Verification items for the finished model (mm, model axes). A direction names the side the tool comes from. Give positions to 0.01 mm unless a question says otherwise; leave off trailing zeros. Loops run counter-clockwise (first coordinate to the right, second up) from the corner with the lowest first, then second, coordinate; pieces in that order, holes last. Notation, with made-up numbers: (64, 9) - (120, 9) arc R15 cw to (120, 36) - close; hole circle Ø8 at (-31.5, -37.5). An arc over 180 degrees is marked (long way). Answer in a Markdown table with one row per item.
```python
from build123d import *

# Parameters (mm, degrees)
EXTRUDE_1_DEPTH     = 19
SKETCH_3_W          = 23.2
SKETCH_3_H          = 9
CUT_EXTRUDE_2_DEPTH = 31.8
CUT_EXTRUDE_3_DEPTH = 8
SKETCH_5_W          = 7.5
SKETCH_5_H          = 7.5
CUT_EXTRUDE_4_DEPTH = 31.8
SKETCH_6_R          = 1.4
CUT_EXTRUDE_5_DEPTH = 27
SKETCH_7_R          = 0.75
CUT_EXTRUDE_6_DEPTH = 31.8
FILLET_2_R          = 0.5
FILLET_3_R          = 2
FILLET_4_R          = 0.5


with BuildPart() as part:
    # 草图1 → 凸台-拉伸1 (new body)
    with BuildSketch(Plane(origin=(0, 0, 0), x_dir=(1, 0, 0), z_dir=(0, 1, 0))):
        Polygon((-5.22, 18.4025), (-2.42, 18.4025), (-2.42, -6.5975), (20.78, -6.5975), (20.78, -12.3975), (-5.22, -12.3975), align=None)
    extrude(amount=EXTRUDE_1_DEPTH)

    # 草图3 → 切除-拉伸2 (cut, through all)
    with BuildSketch(Plane.XY.offset(12.3975)):
        with Locations((9.18, 14.5)):
            Rectangle(SKETCH_3_W, SKETCH_3_H)
    extrude(amount=-CUT_EXTRUDE_2_DEPTH, mode=Mode.SUBTRACT)

    # 草图4 → 切除-拉伸3 (cut)
    with BuildSketch(Plane(origin=(0, 10, 0), x_dir=(1, 0, 0), z_dir=(0, 1, 0))):
        with BuildLine():
            Line((-0.82, -8.4975), (19.18, -8.4975))
            ThreePointArc((19.18, -8.4975), (20.18, -9.4975), (19.18, -10.4975))
            Line((19.18, -10.4975), (-0.82, -10.4975))
            ThreePointArc((-0.82, -10.4975), (-1.82, -9.4975), (-0.82, -8.4975))
        make_face()
    extrude(amount=-CUT_EXTRUDE_3_DEPTH, mode=Mode.SUBTRACT)

    # 草图5 → 切除-拉伸4 (cut, through all)
    with BuildSketch(Plane.XY.offset(12.3975)):
        with Locations((9.18, 6.25)):
            Rectangle(SKETCH_5_W, SKETCH_5_H)
    extrude(amount=-CUT_EXTRUDE_4_DEPTH, mode=Mode.SUBTRACT)

    # 草图6 → 切除-拉伸5 (cut, through all)
    with BuildSketch(Plane.ZY.offset(5.22)):
        with Locations((-16.4025, 17)):
            Circle(SKETCH_6_R)
        with Locations((4.5975, 17)):
            Circle(SKETCH_6_R)
        with Locations((-16.4025, 3.5)):
            Circle(SKETCH_6_R)
        with Locations((4.5975, 3.5)):
            Circle(SKETCH_6_R)
    extrude(amount=-CUT_EXTRUDE_5_DEPTH, mode=Mode.SUBTRACT)

    # 草图7 → 切除-拉伸6 (cut, through all)
    with BuildSketch(Plane.XY.offset(12.3975)):
        with Locations((2.88, 6.2)):
            Circle(SKETCH_7_R)
        with Locations((15.48, 6.2)):
            Circle(SKETCH_7_R)
    extrude(amount=-CUT_EXTRUDE_6_DEPTH, mode=Mode.SUBTRACT)

    # 圆角2
    fillet_2_edges = [part.edges().sort_by_distance(p)[0] for p in [
        (-5.22, 9.5, -18.4025),
        (-2.42, 9.5, -18.4025),
        (-5.22, 9.5, 12.3975),
    ]]
    fillet(fillet_2_edges, radius=FILLET_2_R)

    # 圆角3
    fillet_3_edges = [part.edges().sort_by_distance(p)[0] for p in [
        (20.78, 5, 6.5975),
        (20.78, 5, 12.3975),
    ]]
    fillet(fillet_3_edges, radius=FILLET_3_R)

    # 圆角4
    fillet_4_edges = [part.edges().sort_by_distance(p)[0] for p in [
        (-2.42, 14.5, 12.3975),
    ]]
    fillet(fillet_4_edges, radius=FILLET_4_R)


solid = part.part
```
Q1. Sectioned sample at D-D (z = 4). Record the cut outline in (x, y).
Completed:
| item | result |
|---|---|
| outline | (-5.22, 0) - (-2.42, 0) - (-2.42, 2.23) - (-5.22, 2.23) - close; (-5.22, 4.77) - (-2.42, 4.77) - (-2.42, 15.73) - (-5.22, 15.73) - close; (-5.22, 18.27) - (-2.42, 18.27) - (-2.42, 19) - (-5.22, 19) - close |
Q2. Go/stop test with flat-tipped pins: P1, Ø10, axis at x = 8, y = 9.5, coming from the -Z side; P2, Ø1, axis at x = 7.5, z = 8, coming from the +Y side; P3, Ø2, axis at x = 15.48, y = 6.2, coming from the +Z side; P4, Ø12, axis at x = 11.5, z = 8.5, coming from the +Y side. Record where each tip stops, or that it passes through.
Completed:
| item | result |
|---|---|
| P1 | z = 6.6 |
| P2 | y = 2.5 |
| P3 | z = 12.4 |
| P4 | y = 10 |
Q3. Sectioned sample at A-A (y = 3.5). Give the number of separate pieces and of enclosed holes in the cut face, and give its area (3 significant figures).
Completed:
| item | result |
|---|---|
| separate pieces | 4 |
| enclosed holes | 0 |
| area | 132 mm^2 |
Q4. Tool access check on faces 5 (the face through (8, 2, 6.598)), 6 (the face through (20.18, 6.06, 9.48)), 7 (the face through (9, 2.5, 11)). Record the directions out of +Z, -Z, +X, -X, +Y, -Y that give a thin tool (end or side, any length) a straight path to the whole face; none if there is none.
Completed:
| item | result |
|---|---|
| face 5 | -Z, +X, +Y, -Y |
| face 6 | +Y |
| face 7 | +Z, -Z, +Y |
Q5. Sectioned sample at C-C (x = 15.48). Record the cut outline in (y, z), and give its area (3 significant figures).
Completed:
| item | result |
|---|---|
| outline | (0, 6.6) - (5.45, 6.6) - (5.45, 8.5) - (2, 8.5) - (2, 10.5) - (5.45, 10.5) - (5.45, 12.4) - (0, 12.4) - close; (6.95, 6.6) - (10, 6.6) - (10, 8.5) - (6.95, 8.5) - close; (6.95, 10.5) - (10, 10.5) - (10, 12.4) - (6.95, 12.4) - close |
| area | 36.3 mm^2 |
Q6. Sectioned sample at B-B (y = 8). Record the cut outline in (x, z).
Completed:
| item | result |
|---|---|
| outline | (-5.22, -17.9) arc R0.5 ccw to (-4.72, -18.4) - (-2.92, -18.4) arc R0.5 ccw to (-2.42, -17.9) - (-2.42, 6.6) - (5.43, 6.6) - (5.43, 8.5) - (-0.82, 8.5) arc R1 cw to (-0.82, 10.5) - (5.43, 10.5) - (5.43, 12.4) - (-4.72, 12.4) arc R0.5 ccw to (-5.22, 11.9) - close; (12.93, 6.6) - (18.78, 6.6) arc R2 ccw to (20.78, 8.6) - (20.78, 10.4) arc R2 ccw to (18.78, 12.4) - (12.93, 12.4) - (12.93, 10.5) - (19.18, 10.5) arc R1 cw to (19.18, 8.5) - (12.93, 8.5) - close |
Q7. Thickness scan on line 1 (Y direction, x = 2.88, z = 7.8); line 2 (Z direction, x = 17.25, y = 8); line 3 (X direction, y = 6.25, z = -15.5). Record the ranges inside material, lowest first.
Completed:
| item | result |
|---|---|
| line 1 | 0 to 5.45, 6.95 to 10 |
| line 2 | 6.6 to 8.5, 10.5 to 12.4 |
| line 3 | -5.22 to -2.42 |
Q8. Draft check along Y on faces 1 (the face through (14.73, 6.23, 7.56)), 2 (the face through (-4, 19, -3)), 3 (the face through (20.18, 5.07, 7.17)), 4 (the face through (-3.84, 18.18, 5.35)). Enter one of: +Y half, -Y half, draft (parallel to the pull), parting line (faces both ways), or undercut.
Completed:
| item | result |
|---|---|
| face 1 | undercut |
| face 2 | +Y half |
| face 3 | draft |
| face 4 | undercut |
